Could you check a few things on this model? Use its own coordinates, in mm. A direction names the side the tool comes from. Give positions to 0.01 mm unless a question says otherwise; leave off trailing zeros. Write each loop counter-clockwise with the first axis right and the second up, starting at its lowest first coordinate (ties: lowest second). Pieces come first, ordered by that corner, then holes. Notation, with made-up numbers: M 32,-35 L 79,-35 A9 cw 79,-25 Z; hole C -39.5,-12 d8. An arc over 180 degrees is marked long. One line per item, written item: value.
```python
from build123d import *

# Parameters (mm, degrees)
UBODY_START         = -0.1
UBODY_SKETCH_R      = 5.025
UBODY_DEPTH         = 0.1
NUT_DEPTH           = 11.99
THREAD_CHAMFER_SIZE = 0.25
UTUBE_START         = -13.3
UTUBE_SKETCH_R      = 3.175
UTUBE_DEPTH         = 13.3
UTUBE_RADIUS_R      = 0.5
PORT_SKETCH_R       = 1.984375
PORT_DEPTH          = 22.243724564


with BuildPart() as part:
    # URelease_Sketch → URelease (revolve)
    with BuildSketch(Plane.XY, mode=Mode.PRIVATE) as urelease_sk:
        with BuildLine():
            Line((0, 0), (-4.525, 0))
            ThreePointArc((-4.525, 0), (-4.878553391, -0.146446609), (-5.025, -0.5))
            Line((-5.025, -0.5), (-5.025, -1.5))
            Line((-5.025, -1.5), (-3.575, -1.5))
            Line((-3.575, -1.5), (-3.575, -2.4))
            Line((-3.575, -2.4), (0, -2.4))
            Line((0, -2.4), (0, 0))
        make_face()
    revolve(urelease_sk.sketch.rotate(Axis((0, 0, 0), (0, -1, 0)), 270), axis=Axis((0, 0, 0), (0, -1, 0)))

    # UBody_Sketch → UBody (add)
    with BuildSketch(Plane(origin=(0, -2.4, 0), x_dir=(-1, 0, 0), z_dir=(0, 1, 0)).offset(UBODY_START)):
        with Locations(Location((0, 0, 0), (0, 0, 90))):
            Circle(UBODY_SKETCH_R)
    extrude(amount=UBODY_DEPTH)

    # Nut_Sketch → Nut (add)
    with BuildSketch(Plane(origin=(0, -2.5, 0), x_dir=(-1, 0, 0), z_dir=(0, 1, 0))):
        Polygon((-3.666174209, -6.35), (3.666174209, -6.35), (7.332348419, 0), (3.666174209, 6.35), (-3.666174209, 6.35), (-7.332348419, 0), align=None)
    extrude(amount=-NUT_DEPTH)

    # Nut_Chamfer_Sketch → Nut_Chamfer (revolve, cut)
    with BuildSketch(Plane(origin=(0, 0, 0), x_dir=(0, 0, -1), z_dir=(1, 0, 0))):
        Polygon((-6.35, -2.5), (-9.35, -2.5), (-9.35, -4.232050808), align=None)
        Polygon((-9.35, -12.757949192), (-9.35, -14.49), (-6.35, -14.49), align=None)
    revolve(axis=Axis((0, 0, 0), (0, -1, 0)), mode=Mode.SUBTRACT)

    # Threads_Sketch → Threads (revolve)
    with BuildSketch(Plane.XY, mode=Mode.PRIVATE) as threads_sk:
        Polygon((-4.7715, -15.35), (-4.3, -15.35), (-4.3, -14.49), (0, -14.49), (0, -18.9), (-4.7715, -18.9), align=None)
    revolve(threads_sk.sketch.rotate(Axis((0, 0, 0), (0, -1, 0)), 270), axis=Axis((0, 0, 0), (0, -1, 0)))

    # Thread_Chamfer
    thread_chamfer_edges = [part.edges().sort_by_distance(p)[0] for p in [
        (0, -18.9, -4.7715),
        (0, -15.35, -4.7715),
    ]]
    chamfer(thread_chamfer_edges, length=THREAD_CHAMFER_SIZE)

    # UTube_Sketch → UTube (cut)
    with BuildSketch(Plane(origin=(0, 0, 0), x_dir=(1, 0, 0), z_dir=(0, 1, 0)).offset(UTUBE_START)):
        with Locations(Location((0, 0, 0), (0, 0, 270))):
            Circle(UTUBE_SKETCH_R)
    extrude(amount=UTUBE_DEPTH, mode=Mode.SUBTRACT)

    # UTube_Radius
    utube_radius_edges = [part.edges().sort_by_distance(p)[0] for p in [
        (0, 0, -3.175),
    ]]
    fillet(utube_radius_edges, radius=UTUBE_RADIUS_R)

    # Port_Sketch → Port (cut, through all)
    with BuildSketch(Plane(origin=(0, 0, 0), x_dir=(1, 0, 0), z_dir=(0, 1, 0))):
        with Locations(Location((0, 0, 0), (0, 0, 270))):
            Circle(PORT_SKETCH_R)
    extrude(amount=-PORT_DEPTH, mode=Mode.SUBTRACT)

    # Sketch1 → Cut-Revolve2 (revolve, cut)
    with BuildSketch(Plane.XY, mode=Mode.PRIVATE) as cut_revolve2_sk:
        Polygon((-4.3, -14.49), (-7.332348419, -11.457651581), (-7.332348419, -14.49), align=None)
    revolve(cut_revolve2_sk.sketch.rotate(Axis((0, -18.9, 0), (0, 1, 0)), 270), axis=Axis((0, -18.9, 0), (0, 1, 0)), mode=Mode.SUBTRACT)


solid = part.part
```
1) We'd pull the mould along Z, two halves only. Please class faces 4 (the face through (-1.93, -6.99, -2.52)), 5 (the face through (4.383, -14.3, 0.973)), 6 (the face through (5.474, -7.4, 3.219)): pulls with the +Z half, pulls with the -Z half, needs draft (parallel to the pull), parting line crosses it, or undercut.
Outcome:
face 4: undercut
face 5: parting line crosses it
face 6: pulls with the +Z half
2) If we section it at A-A, the plane y = -8.5: Write out the boundary of the cut face in (x, z) (3 decimals).
Outcome:
outline: M -7.332,0 L -3.666,-6.35 L 3.666,-6.35 L 7.332,0 L 3.666,6.35 L -3.666,6.35 Z; hole C 0,0 d6.35
3) I'm going to push flat-ended pins straight in: pin 1 (8 mm diameter, centred on x = 2.5, y = -12.5, fed in from +Z); pin 2 (2.5 mm diameter, centred on x = -1.5, z = 0.5, fed in from +Y); pin 3 (3 mm diameter, centred on y = -8, z = -3.5, fed in from -X); pin 4 (1 mm diameter, centred on y = -16, z = 0.5, fed in from -X). Where does each tip first touch, or does it pass through?
Outcome:
pin 1: stops at z = 6.35
pin 2: stops at y = -13.3
pin 3: stops at x = -6.18
pin 4: stops at x = -4.77
4) Please list where these lines run through material, in increasing order: L1, parallel to Y at x = 4.25, z = 2; L2, parallel to X at y = -17.45, z = 0; L3, parallel to Y at x = -2.75, z = -2.75. Write a range as from..to.
Outcome:
L1: y = -18.72..-15.53, -14.09..-2.4, -1.5..-0.03
L2: x = -4.77..-1.98, 1.98..4.77
L3: y = -18.9..-2.4, -1.5..0
5) On a 3-axis mill with a long thin cutter (end or side, diameter ignored), from which of +Z, -Z, +X, -X, +Y, -Y can I reach the whole of each face in a straight line? I mean faces 1 (the face through (-2, -13.3, 1)), 2 (the face through (3.306, -2.635, 5.694)), 3 (the face through (-3.545, -1.956, -0.465)). Say none if no direction works.
Outcome:
face 1: +Y
face 2: +Z, +X, +Y
face 3: none
6) If we section it at C-C, the plane y = -17.25: Write out the boundary of the cut face in (x, z), then the cut area to 3 significant figures.
Outcome:
outline: C 0,0 d9.54; hole C 0,0 d3.97
area: 59.2 mm^2
7) If we section it at B-B, the plane y = -14.25: Write out the boundary of the cut face in (x, z), then the cut area to 3 significant figures.
Outcome:
outline: C 0,0 d9.08; hole C 0,0 d3.97
area: 52.4 mm^2
